Solid Edge part; units mm, degrees
sketch "Sketch1" plane through (0, 0, 0) normal (0, -1, 0) x (1, 0, 0)
  line L0 (-50, 0) -> (0, 0)
  line L1 (0, 0) -> (0, 2)
  line L2 (0, 2) -> (15, 2)
  line L3 (15, 2) -> (15, 0)
  line L4 (15, 0) -> (17, 0)
  line L5 (17, 0) -> (17, 5)
  line L6 (17, 5) -> (-50, 5)
  line L7 (-50, 5) -> (-50, 0)
  dimension "D1" = 17
  dimension "D2" = 15
  dimension "D3" = 50
extrude "Protrusion1" add sketch "Sketch1" against normal blind 50
hole "Agujero_1" at (7.5, 10, 5) direction (0, 0, -1) diameter 6.4 end up to next countersink diameter 13.71 countersink angle 90
hole "Hole1" at (7.5, 25, 5) direction (0, 0, -1) diameter 6.4 end up to next countersink diameter 13.71 countersink angle 90
hole "Hole2" at (7.5, 40, 5) direction (0, 0, -1) diameter 6.4 end up to next countersink diameter 13.71 countersink angle 90
sketch "Sketch2" plane through (-25, 25, 0) normal (0, 0, -1) x (-1, 0, 0)
  circle A0 centre (-1.5, -13.5) radius 1.25
  circle A1 centre (6.5, -13.5) radius 1.25
  circle A2 centre (14.5, -13.5) radius 1.25
  circle A3 centre (20, -8) radius 1.25
  circle A4 centre (20, 8) radius 1.25
  circle A5 centre (14.5, 13.5) radius 1.25
  circle A6 centre (-1.5, 13.5) radius 1.25
  circle A7 centre (6.5, 13.5) radius 1.25
  circle A8 centre (-9.5, 13.5) radius 1.25
  circle A9 centre (-9.5, -13.5) radius 1.25
extrude "Cutout1" cut sketch "Sketch2" against normal up to next
sketch "Sketch3" plane through (-16.5, 25, 5) normal (0, 0, 1) x (1, 0, 0)
  line L0 (-25.5, -11) -> (14.5, -11)
  line L1 (14.5, -11) -> (14.5, 11)
  line L2 (14.5, 11) -> (-25.5, 11)
  line L3 (-25.5, 11) -> (-25.5, -11)
  dimension "D1" = 14.5
  dimension "D2" = 14.5
extrude "Cutout2" cut sketch "Sketch3" against normal up to next
fillet "Redondeo_1" radius 3 4 edges at (-42, 36, 2.5) (-42, 14, 2.5) (-2, 14, 2.5) (-2, 36, 2.5)
properties part number "1976-1400-002" material "Aluminio, 7075-T6"
Work out the finished part from the listing and answer in its coordinate system (mm). A direction names the side the tool comes from. Give positions to 0.01 mm unless a question says otherwise; leave off trailing zeros. Order: outer loops, then holes, each group sorted by start corner. A loop starts at its lowest first (then second) coordinate and runs counter-clockwise, first axis right, second up. Notation, with made-up numbers: M 34,27.25 L 78,27.25 A19 cw 78,43.25 Z; hole C 23.25,26.5 d2. An arc over 180 degrees is marked long. Return JSON: item names as keys, results as strings.
1) A tool of negligible diameter and unlimited length cuts with its end or side. For faces 1 (the flat face through (15, 25, 1)), 2 (the flat face through (-22, 14, 3)), 3 (the flat face through (-25.3, 13.5, 0)), from which of +Z, -Z, +X, -X, +Y, -Y can it reach the whole face along a straight path? Write none if from no direction.
Resolved:
{"face 1": "-Z, +Y, -Y", "face 2": "+Z, -Z", "face 3": "-Z, +X, -X, +Y, -Y"}
2) Section D-D, the plane y = 25 is taken. Write down the section's boundary in (x, z) (3 decimals), plus the area to 3 significant figures.
Resolved:
{"outline": "M -50,0 L -42,0 L -42,5 L -50,5 Z; M -2,0 L 0,0 L 0,2 L 3.645,2 L 0.645,5 L -2,5 Z; M 11.355,2 L 15,2 L 15,0 L 17,0 L 17,5 L 14.355,5 Z", "area": "72.9 mm^2"}
3) Section A-A, the plane x = -6 is taken. Write down the section's boundary in (y, z).
Resolved:
{"outline": "M 0,0 L 14,0 L 14,5 L 0,5 Z; M 36,0 L 50,0 L 50,5 L 36,5 Z"}
4) For a pull along Y with two mould halves and no side action, classify faces 4 (the flat face through (-16, 50, 3)), 5 (the cylindrical face through (-2.9, 35.14, 2.46)), 6 (the flat face through (16, 25, 0)), 7 (the cylindrical face through (-24.655, 38.021, 2.465)) as +Y half, -Y half, draft (parallel to the pull), parting line (faces both ways), or undercut.
Resolved:
{"face 4": "+Y half", "face 5": "undercut", "face 6": "draft", "face 7": "undercut"}
5) Straight lines are drawn through the part: line 1 along Y through (x, z) = (-31.5, 2); line 2 along X through (y, z) = (37, 1.75); line 3 along Y through (x, z) = (-45, 2). For each, find the intervals that lie inside material, in ascending order. Write a range as [from, to].
Resolved:
{"line 1": "[0, 10.25], [12.75, 14], [36, 37.25], [39.75, 50]", "line 2": "[-50, 0], [15, 17]", "line 3": "[0, 15.75], [18.25, 31.75], [34.25, 50]"}
6) Section B-B, the plane x = -15.5 is taken. Write down the section's boundary in (y, z), plus the area to 3 significant figures.
Resolved:
{"outline": "M 0,0 L 10.25,0 L 10.25,5 L 0,5 Z; M 12.75,0 L 14,0 L 14,5 L 12.75,5 Z; M 36,0 L 37.25,0 L 37.25,5 L 36,5 Z; M 39.75,0 L 50,0 L 50,5 L 39.75,5 Z", "area": "115 mm^2"}
7) Each of these flat-tipped pins is pushed along its axis until it touches: pin 1 (2 mm diameter, centred on x = -31.5, y = 11.5, fed in from +Z); pin 2 (12 mm diameter, centred on x = 6.5, y = 10.5, fed in from -Z). Where does it stop, or does it pass through?
Resolved:
{"pin 1": "through", "pin 2": "z = 2"}
8) Section C-C, the plane z = 3.3 is taken. Give the number of separate pieces and of enclosed holes in the cut face, plus the area to 3 significant figures.
Resolved:
{"separate pieces": "1", "enclosed holes": "14", "area": "2,180 mm^2"}
